from build123d import *

# Parameters (mm, degrees)
F0_R     = 1.425
F0_R_2   = 1.575
F1_DEPTH = 4
F3_DEPTH = 1.5
F4_R     = 3.138478
F0_W     = 2
F0_H     = 7.5
F0_W_2   = 10.5
F5_DEPTH = 4
F6_DEPTH = 15.5
F7_R     = 1
F8_DEPTH = 3
F9_R     = 2


with BuildPart() as f1:
    # F0 (on Front) → F1 (new body)
    with BuildSketch(Plane.XZ):
        Polygon((5, 13.5), (-13.5, 13.5), (-13.5, 0), (-13.5, -7.5), (5, -7.5), align=None)
        with Locations((-8.5, -2.5)):
            Circle(F0_R, mode=Mode.SUBTRACT)
        with Locations((0, -2.5)):
            Circle(F0_R, mode=Mode.SUBTRACT)
        with Locations((-8.5, 8.5)):
            Circle(F0_R_2, mode=Mode.SUBTRACT)
        with Locations((0, 8.5)):
            Circle(F0_R_2, mode=Mode.SUBTRACT)
    extrude(amount=-F1_DEPTH)

    # F2 (on face) → F3 (cut)
    with BuildSketch(Plane(origin=(0, 4, 0), x_dir=(-1, 0, 0), z_dir=(0, 1, 0))):
        Polygon((-0.699741, 5.373043), (2.358154, 6.330527), (3.057895, 9.457485), (0.699741, 11.626957), (-2.358154, 10.669473), (-3.057895, 7.542515), align=None)
        Polygon((7.800259, 5.373043), (10.858154, 6.330527), (11.557895, 9.457485), (9.199741, 11.626957), (6.141846, 10.669473), (5.442105, 7.542515), align=None)
    extrude(amount=-F3_DEPTH, mode=Mode.SUBTRACT)

    # F4
    f4_edges = [f1.edges().sort_by_distance(p)[0] for p in [
        (5, 2, 13.5),
        (-13.5, 2, 13.5),
        (5, 2, -7.5),
    ]]
    fillet(f4_edges, radius=F4_R)

    # F0 (on Front) → F5 (join)
    with BuildSketch(Plane.XZ):
        with Locations((-25, -3.75)):
            Rectangle(F0_W, F0_H)
        with Locations((-18.75, -3.75)):
            Rectangle(F0_W_2, F0_H)
    extrude(amount=-F5_DEPTH)

    # F0 (on Front) → F6 (join)
    with BuildSketch(Plane.XZ):
        with Locations((-25, -3.75)):
            Rectangle(F0_W, F0_H)
    extrude(amount=-F6_DEPTH)

    # F7 (on face) → F8 (cut)
    with BuildSketch(Plane(origin=(-26, 0, 0), x_dir=(0, -1, 0), z_dir=(-1, 0, 0))):
        with Locations((-13.5, -3)):
            Circle(F7_R)
        with Locations((-7.3, -3)):
            Circle(F7_R)
    extrude(amount=-F8_DEPTH, mode=Mode.SUBTRACT)

    # F9
    f9_edges = [f1.edges().sort_by_distance(p)[0] for p in [
        (-24, 4, -3.75),
    ]]
    fillet(f9_edges, radius=F9_R)


solid = f1.part
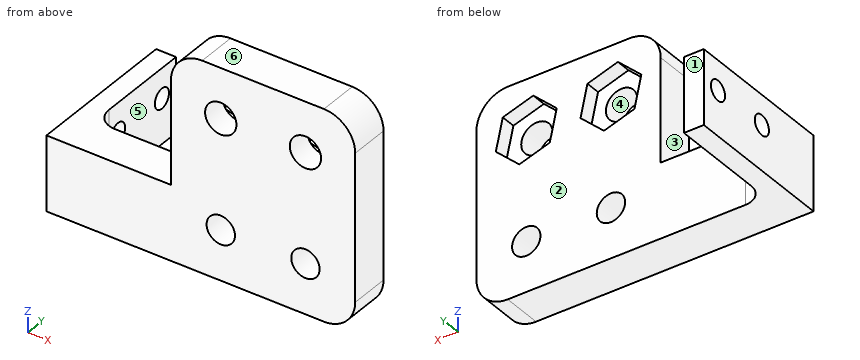
Here's how the part is built. I have some questions about the finished solid (model axes, mm). Face numbers are marked on the shaded views. A direction names the side the tool comes from. Coordinates: 2 decimals unless noted, no trailing zeros. Loops run counter-clockwise (first coordinate to the right, second up) from the corner with the lowest first, then second, coordinate; pieces in that order, holes last.
1. Imagine slicing it at A-A, the plane y = 7.3. Please give me the cut outline in (x, z), and give its area (3 significant figures).
2. Imagine slicing it at D-D, the plane x = -19.5. Please give me the cut outline in (y, z), and give its area (3 significant figures).
3. If we mould it in two halves opening along Z, with no side actions, what happens to the marked faces 4, 5 and 6? For each: pulls with the +Z half, pulls with the -Z half, needs draft (parallel to the pull), parting line crosses it, or undercut.
4. Imagine slicing it at C-C, the plane z = 3. Please give me the cut outline in (x, y), and give its area (3 significant figures).
5. I need wall thicknesses on L1, parallel to Z at x = -8.5, y = 1.4 (3 decimals); L2, parallel to Z at x = -25.2, y = 13.5; L3, parallel to Y at x = -20, z = -5. Which ranges of each line are inside material? Lowest first, please.
6. For P1, Ø1.8, axis at x = -10, z = 9.5, coming from the +Y side; P2, Ø1, axis at x = -3, z = -0.5, coming from the +Y side; P3, Ø1.7, axis at x = 0, z = -2.5, coming from the +Y side; P4, Ø2, axis at y = 2.5, z = 7, coming from the -X side, each with a flat end and sliding along its axis, tell me the tip position at first contact or that it passes through.
7. For the marked faces 1, 2 and 3, which set-ups out of +Z, -Z, +X, -X, +Y, -Y let a thin tool reach every point of the face, with its end or its side?
8. Imagine slicing it at B-B, the plane x = -8.5. Please give me the cut outline in (y, z) (3 decimals), and give its area (3 significant figures).
Taken from the geometry:
1. outline: (-26, -7.5) - (-24, -7.5) - (-24, -4) - (-26, -4) - close; (-26, -2) - (-24, -2) - (-24, 0) - (-26, 0) - close
1. area: 11.0 mm2
2. outline: (0, -7.5) - (4, -7.5) - (4, 0) - (0, 0) - close
2. area: 30.0 mm2
3. face 4: undercut
3. face 5: needs draft
3. face 6: pulls with the +Z half
4. outline: (-13.5, 0) - (5, 0) - (5, 4) - (-13.5, 4) - close
4. area: 74.0 mm2
5. L1: z = -7.5 to -3.925, -1.075 to 6.925, 10.075 to 13.5
5. L2: z = -7.5 to -4, -2 to 0
5. L3: y = 0 to 4
6. P1: stops at y = 2.5
6. P2: stops at y = 4
6. P3: passes through
6. P4: stops at x = -13.5
7. face 1: +Z, -Z, +X, -X, +Y
7. face 2: +Z, -Z, +X, +Y
7. face 3: +Z, -X, +Y, -Y
8. outline: (0, -7.5) - (4, -7.5) - (4, -3.925) - (0, -3.925) - close; (0, -1.075) - (4, -1.075) - (4, 5.592) - (2.5, 5.592) - (2.5, 6.925) - (0, 6.925) - close; (0, 10.075) - (2.5, 10.075) - (2.5, 11.408) - (4, 11.408) - (4, 13.5) - (0, 13.5) - close
8. area: 56.0 mm2
